```python
from build123d import *

# Parameters (mm, degrees)
EXTRUDE_1_DEPTH          = 25.6
EXTRUDE_1_DEPTH_BACK     = 1000
SKETCH_1_R               = 10
CUT_EXTRUDE_1_DEPTH      = 1001.530359359
CUT_EXTRUDE_1_DEPTH_BACK = 1001.530359359
SKETCH_2_R               = 4.1
CHAMFER_1_SIZE           = 1


with BuildPart() as part:
    # Эскиз1 → Бобышка-Вытянуть1 (new, two sides: drawn at the far end of the back side and taken through both)
    with BuildSketch(Plane.XY.offset(-EXTRUDE_1_DEPTH_BACK)):
        with Locations((21, 0)):
            Circle(SKETCH_1_R)
    extrude(amount=EXTRUDE_1_DEPTH + EXTRUDE_1_DEPTH_BACK)

    # Эскиз2 → Вырез-Вытянуть1 (cut, two sides: drawn at the far end of the back side and taken through both)
    with BuildSketch(Plane(origin=(0, 0, 0), x_dir=(0, 0, -1), z_dir=(1, 0, 0)).offset(-CUT_EXTRUDE_1_DEPTH_BACK)):
        with Locations(Location((-14, 0, 0), (0, 0, 180))):
            Circle(SKETCH_2_R)
    extrude(amount=CUT_EXTRUDE_1_DEPTH + CUT_EXTRUDE_1_DEPTH_BACK, mode=Mode.SUBTRACT)

    # Фаска1
    chamfer_1_edges = [part.edges().sort_by_distance(p)[0] for p in [
        (11, 0, 25.6),
    ]]
    chamfer(chamfer_1_edges, length=CHAMFER_1_SIZE)


solid = part.part
```
Design review of the part built by this model. Coordinates are the model's own, in mm. Coordinates: 2 decimals unless noted, no trailing zeros. Order: outer loops, then holes, each group sorted by start corner. A loop starts at its lowest first (then second) coordinate and runs counter-clockwise, first axis right, second up. Notation, with made-up numbers: M -39.75,82 L 13.25,82 A16 cw 13.25,87 Z; hole C 58.25,71 d11. An arc over 180 degrees is marked long. Answer as a JSON object with one key per item and string values. Group by question number.
1) Wall thickness on L1, parallel to Y at x = 25.25, z = 14; L2, parallel to Z at x = 23.75, y = -0.5; L3, parallel to Y at x = 25, z = 14: over which ranges is each line inside the solid? List them lowest first.
2) For pin 1 (1.5 mm diameter, centred on x = 14, z = -784.5, fed in from +Y); pin 2 (5 mm diameter, centred on x = 14.5, z = -789, fed in from +Y); pin 3 (3 mm diameter, centred on y = 4.5, z = -518.5, fed in from +X), all flat-tipped, find the tip position at first contact; note any pin that passes through.
3) Add section A-A, the plane z = -396. Write out the cut boundary in (x, y), then the cut area to 3 significant figures.
Computed values:
{
 "1": {"L1": "y = -9.05 to -4.1, 4.1 to 9.05", "L2": "z = -1000 to 9.93, 18.07 to 25.6", "L3": "y = -9.17 to -4.1, 4.1 to 9.17"},
 "2": {"pin 1": "stops at y = 7.81", "pin 2": "stops at y = 9.17", "pin 3": "stops at x = 30.54"},
 "3": {"outline": "C 21,0 d20", "area": "314 mm^2"}
}
